```python
from build123d import *

# Parameters (mm, degrees)
CYLINDER004_R          = 10
CYLINDER004_DEPTH      = 10
CYLINDER003_R          = 11.3
CYLINDER003_DEPTH      = 2
CYLINDER002_R          = 4
CYLINDER002_DEPTH      = 40
CYLINDER002_ROLL_ANGLE = 90
CYLINDER001_R          = 11.2
CYLINDER001_DEPTH      = 16
CYLINDER_R             = 20
CYLINDER_DEPTH         = 16


with BuildPart() as cylinder004:
    # Cylinder004 → Cylinder004 (new body)
    with BuildSketch(Plane(origin=(5, 0, 0), x_dir=(1, 0, 0), z_dir=(0, 0, 1))):
        Circle(CYLINDER004_R)
    extrude(amount=CYLINDER004_DEPTH)


with BuildPart() as cylinder003:
    # Cylinder003 → Cylinder003 (new body)
    with BuildSketch(Plane(origin=(5, 0, 7), x_dir=(1, 0, 0), z_dir=(0, 0, 1))):
        Circle(CYLINDER003_R)
    extrude(amount=CYLINDER003_DEPTH)


with BuildPart() as cylinder002:
    # Cylinder002 → Cylinder002 (new body)
    with BuildSketch(Plane.XY):
        Circle(CYLINDER002_R)
    extrude(amount=CYLINDER002_DEPTH)


with BuildPart() as cylinder002_1:
    # Cylinder002 roll: moved
    add(cylinder002.part.rotate(Axis((0, 0, 0), (1, 0, 0)), CYLINDER002_ROLL_ANGLE))


with BuildPart() as cylinder002_2:
    # Cylinder002 placement: moved
    add(cylinder002_1.part.moved(Location((-10, 26, 8))))


with BuildPart() as cylinder001:
    # Cylinder001 → Cylinder001 (new body)
    with BuildSketch(Plane(origin=(5, 0, 0), x_dir=(1, 0, 0), z_dir=(0, 0, 1))):
        Circle(CYLINDER001_R)
    extrude(amount=CYLINDER001_DEPTH)


with BuildPart() as cut002:
    # Cylinder → Cylinder (new body)
    with BuildSketch(Plane.XY):
        Circle(CYLINDER_R)
    extrude(amount=CYLINDER_DEPTH)

    # Cut: cut Cylinder001
    add(cylinder001.part, mode=Mode.SUBTRACT)

    # Cut001: cut Cylinder002
    add(cylinder002_2.part, mode=Mode.SUBTRACT)

    # Fusion: union Cylinder003
    add(cylinder003.part)

    # Cut002: cut Cylinder004
    add(cylinder004.part, mode=Mode.SUBTRACT)


solid = cut002.part
```
Input: part model. Units: mm. Frame: model coordinates. A direction names the side the tool comes from. Give positions to 0.01 mm unless a question says otherwise; leave off trailing zeros. Order: outer loops, then holes, each group sorted by start corner. A loop starts at its lowest first (then second) coordinate and runs counter-clockwise, first axis right, second up. Notation, with made-up numbers: (14, -21) - (26, -21) arc R18 ccw to (26, -10) - close; hole circle Ø4 at (27.25, 39.5). An arc over 180 degrees is marked (long way). One line per item, written item: value.
1. Reachability of faces 1 (the face through (-6.19, 0.49, 3.45)), 2 (the face through (-6.19, 0.49, 12.45)), 3 (the face through (14.54, 3, 7.99)) from +Z, -Z, +X, -X, +Y, -Y: full face, straight path, thin tool, end or side. Return the list, or none.
Determined:
face 1: -Z
face 2: +Z
face 3: +Z, -Z
2. Cut plane A-A, the plane y = 12. Output: boundary loops of the cut face in (x, z).
Determined:
outline: (-16, 0) - (16, 0) - (16, 16) - (-16, 16) - close; hole circle Ø8 at (-10, 8)
3. Pin query (flat end, axial travel): pin 1 Ø11 at (x, y) = (0, -4.5) entering from -Z; pin 2 Ø5 at (y, z) = (-6.5, 10.5) entering from +X; pin 3 Ø6.5 at (x, z) = (-10, 8) entering from +Y; pin 4 Ø1 at (x, y) = (11.5, 4) entering from +Z. Return the tip coordinate at first contact, or that it passes through.
Determined:
pin 1: z = 0
pin 2: x = 19.6
pin 3: y = -14
pin 4: through
4. Draft query along X for faces 4 (the face through (-4.336, -19.524, 7.888)), 5 (the face through (-6.3, 0, 8)), 6 (the face through (-9, 0, 0)). Return one class per face: released by +X, released by -X, zero draft, split by the parting line, or undercut.
Determined:
face 4: split by the parting line
face 5: undercut
face 6: zero draft
5. Line query: probe 1 along Z at (x, y) = (-10, 14.5); probe 2 along Y at (x, z) = (5, 13); probe 3 along X at (y, z) = (-12.5, 10.5). Output: solid intervals per line, ascending.
Determined:
probe 1: 0 to 4, 12 to 16
probe 2: -19.36 to -11.2, 11.2 to 19.36
probe 3: -15.61 to -13.12, -6.88 to 15.61
6. Cut plane D-D, the plane z = 3.25. Output: boundary loops of the cut face in (x, y), and give its area (3 significant figures).
Determined:
outline: circle Ø40 at (0, 0); hole circle Ø22.4 at (5, 0)
area: 863 mm2
7. Cut plane C-C, the plane y = 0. Output: boundary loops of the cut face in (x, z), and give its area (3 significant figures).
Determined:
outline: (-20, 0) - (-6.2, 0) - (-6.2, 6.75) arc R4 cw (long way) to (-6.2, 9.25) - (-6.2, 16) - (-20, 16) - close; (-6.3, 7) - (-5, 7) - (-5, 9) - (-6.3, 9) - close; (15, 7) - (16.2, 7) - (16.2, 0) - (20, 0) - (20, 16) - (16.2, 16) - (16.2, 9) - (15, 9) - close
area: 237 mm2
8. Cut plane B-B, the plane x = -1.5. Output: boundary loops of the cut face in (y, z).
Determined:
outline: (-19.94, 0) - (-9.12, 0) - (-9.12, 7) - (-7.6, 7) - (-7.6, 9) - (-9.12, 9) - (-9.12, 16) - (-19.94, 16) - close; (7.6, 7) - (9.12, 7) - (9.12, 0) - (19.94, 0) - (19.94, 16) - (9.12, 16) - (9.12, 9) - (7.6, 9) - close
